from build123d import *

# Parameters (mm, degrees)
CUT_EXTRUDE1_START  = -14.5
SKETCH2_R           = 2.5
SKETCH2_R_2         = 2.3
CUT_EXTRUDE1_DEPTH  = 9
BOSS_EXTRUDE2_REACH = 21.818
SKETCH3_R           = 0.15


# Read off the part's stored shape, not the designer's step: Extrude-Thin1
with BuildPart() as part:
    # Extrude-Thin1 outline → Extrude-Thin1 (revolve)
    with BuildSketch(Plane.YX):
        Polygon((2.5, 20), (0, 20), (0, 19.5), (1.5, 19.5), (1.5, 0.5), (0, 0.5), (0, 0), (2.5, 0), align=None)
    revolve(axis=Axis((0, 0, 0), (1, 0, 0)))

    # Sketch2 → Cut-Extrude1 (cut)
    with BuildSketch(Plane.ZY.offset(CUT_EXTRUDE1_START)):
        Circle(SKETCH2_R)
        Circle(SKETCH2_R_2, mode=Mode.SUBTRACT)
    extrude(amount=CUT_EXTRUDE1_DEPTH, mode=Mode.SUBTRACT)

    # Sketch3 → Boss-Extrude2 (add, up to next)
    with BuildSketch(Plane(origin=(0.5, 0, 0), x_dir=(0, 0, -1), z_dir=(1, 0, 0)), mode=Mode.PRIVATE) as boss_extrude2_sk1:
        Circle(SKETCH3_R)
    boss_extrude2_tool1 = extrude(boss_extrude2_sk1.sketch, amount=BOSS_EXTRUDE2_REACH, mode=Mode.PRIVATE) - part.part
    add(boss_extrude2_tool1.solids().sort_by_distance((0.5, 0, 0))[0])


solid = part.part
CAD build for the part. Positions are in the model's coordinates, mm. A direction names the side the tool comes from. Give positions to 0.01 mm unless a question says otherwise; leave off trailing zeros. Loops run counter-clockwise (first coordinate to the right, second up) from the corner with the lowest first, then second, coordinate; pieces in that order, holes last. Notation, with made-up numbers: M 9,29 L 14,29 A21 cw 14,64 Z; hole C 11.5,15.25 d1. An arc over 180 degrees is marked long. Answer in a Markdown table with one row per item. Add a question column.
Item 1: Band-saw the part on A-A on x = 5. Give the cut face in (y, z), then the cut area to 3 significant figures.
Item 2: Tool access for faces 4 (the face through (20, 0, 0)), 5 (the face through (19.5, -0.31, 0.02)): list every direction of +Z, -Z, +X, -X, +Y, -Y with a clear straight run to the whole face (end or side of a thin tool).
Item 3: Band-saw the part on B-B on z = 1.1. Give the cut face in (x, y) (3 decimals), then the cut area to 3 significant figures.
Item 4: Drop flat-ended pins along their axis: P1, Ø1, axis at x = 9, z = 0, coming from the -Y side; P2, Ø1.5, axis at x = 7, y = 1, coming from the -Z side; P3, Ø2, axis at x = 16.5, z = 1.5, coming from the -Y side. Give the stop position or say it passes through.
Item 5: Band-saw the part on C-C on y = 1.7. Give the cut face in (x, z).
Item 6: Probe probe 1 along Z at (x, y) = (5, 0); probe 2 along X at (y, z) = (2.15, 1.15); probe 3 along X at (y, z) = (-0.5, 1.1). List the from-to ranges inside material, lowest first.
Item 7: Mould opens along Y. For faces 1 (the face through (2.79, -0.54, -2.44)), 2 (the face through (0.5, 0.31, 0.02)), 3 (the face through (0, 0, 0)) say: +Y half, -Y half, draft (parallel to the pull), parting line (faces both ways), or undercut.
Item 8: Band-saw the part on D-D on y = -0.5. Give the cut face in (x, z) (3 decimals).
Reply:
| question | item | result |
|---|---|---|
| 1 | outline | C 0,0 d5; C 0,0 d0.3; hole C 0,0 d3 |
| 1 | area | 12.6 mm^2 |
| 2 | face 4 | +Z, -Z, +X, +Y, -Y |
| 2 | face 5 | none |
| 3 | outline | M 0,-2.245 L 5.5,-2.245 L 5.5,-2.02 L 14.5,-2.02 L 14.5,-2.245 L 20,-2.245 L 20,2.245 L 14.5,2.245 L 14.5,2.02 L 5.5,2.02 L 5.5,2.245 L 0,2.245 Z; hole M 0.5,-1.02 L 19.5,-1.02 L 19.5,1.02 L 0.5,1.02 Z |
| 3 | area | 47.0 mm^2 |
| 4 | P1 | stops at y = -2.3 |
| 4 | P2 | stops at z = -2.29 |
| 4 | P3 | stops at y = -2.45 |
| 5 | outline | M 0,-1.83 L 5.5,-1.83 L 5.5,-1.55 L 14.5,-1.55 L 14.5,-1.83 L 20,-1.83 L 20,1.83 L 14.5,1.83 L 14.5,1.55 L 5.5,1.55 L 5.5,1.83 L 0,1.83 Z |
| 6 | probe 1 | z = -2.5 to -1.5, -0.15 to 0.15, 1.5 to 2.5 |
| 6 | probe 2 | x = 0 to 5.5, 14.5 to 20 |
| 6 | probe 3 | x = 0 to 0.5, 19.5 to 20 |
| 7 | face 1 | parting line |
| 7 | face 2 | undercut |
| 7 | face 3 | draft |
| 8 | outline | M 0,-2.449 L 5.5,-2.449 L 5.5,-2.245 L 14.5,-2.245 L 14.5,-2.449 L 20,-2.449 L 20,2.449 L 14.5,2.449 L 14.5,2.245 L 5.5,2.245 L 5.5,2.449 L 0,2.449 Z; hole M 0.5,-1.414 L 19.5,-1.414 L 19.5,1.414 L 0.5,1.414 Z |
